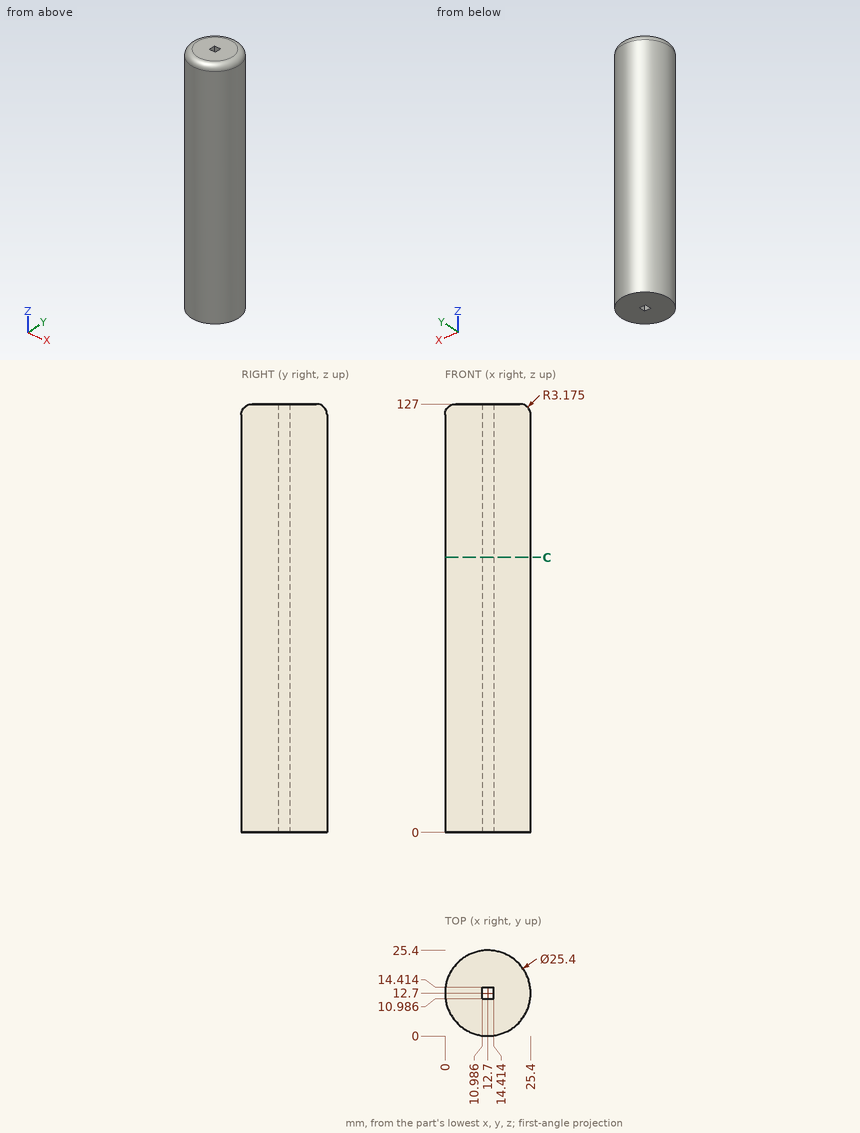
Could you check a few things on this drawing? It's one solid part, dimensions in mm from its lowest x, y, z. Round coordinates to 2 decimals unless told otherwise and drop trailing zeros. Loops run counter-clockwise (first coordinate to the right, second up) from the corner with the lowest first, then second, coordinate; pieces in that order, holes last.
Q1. For P1, Ø1, axis at y = 13.5, z = 75, coming from the -X side; P2, Ø5, axis at x = 17.5, z = 84, coming from the +Y side; P3, Ø10, axis at x = 3.5, z = 37, coming from the -Y side (1 decimal), each with a flat end and sliding along its axis, tell me the tip position at first contact or that it passes through.
Q2. I want a section at C-C (z = 81.5). Write out the boundary of the cut face in (x, y) (1 decimal), and give its area (3 significant figures).
Q3. Please list where these lines run through material, in increasing order: L1, parallel to Y at x = 12, z = 73 (1 decimal); L2, parallel to Y at x = 21.5, z = 90.5 (1 decimal); L3, parallel to X at y = 18, z = 122.
Answer below:
1. P1: stops at x = 0
1. P2: stops at y = 25.19
1. P3: stops at y = 0.7
2. outline: circle Ø25.4 at (12.7, 12.7); hole (11, 11) - (14.4, 11) - (14.4, 14.4) - (11, 14.4) - close
2. area: 495 mm2
3. L1: y = 0 to 11, 14.4 to 25.4
3. L2: y = 3.5 to 21.9
3. L3: x = 1.16 to 24.24
